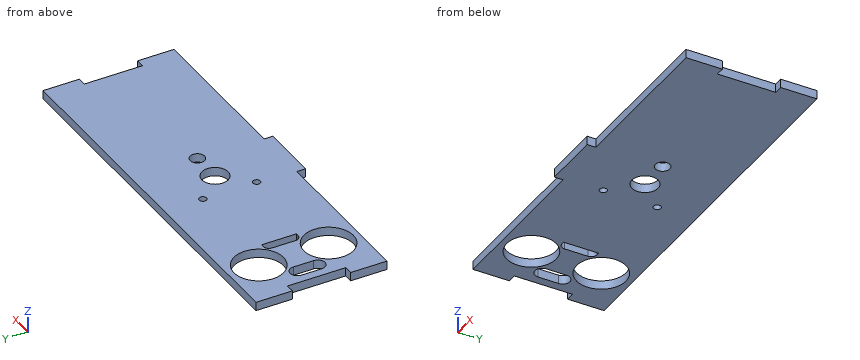
from build123d import *

# Parameters (mm, degrees)
SKETCH1_R           = 8.5
SKETCH1_R_2         = 4.5
SKETCH1_R_3         = 2.5
SKETCH1_R_4         = 1.25
BOSS_EXTRUDE1_DEPTH = 3


with BuildPart() as part:
    # Sketch1 → Boss-Extrude1 (new body)
    with BuildSketch(Plane.XY):
        Polygon((-10, -22.5), (-65, -22.5), (-65, -10), (-62, -10), (-62, 10), (-65, 10), (-65, 22.5), (65, 22.5), (65, 10), (62, 10), (62, -10), (65, -10), (65, -22.5), (10, -22.5), (10, -25.5), (-10, -25.5), align=None)
        with Locations((-48, 12)):
            Circle(SKETCH1_R, mode=Mode.SUBTRACT)
        with Locations((-48, -12)):
            Circle(SKETCH1_R, mode=Mode.SUBTRACT)
        Circle(SKETCH1_R_2, mode=Mode.SUBTRACT)
        with Locations((10.75, 0)):
            Circle(SKETCH1_R_3, mode=Mode.SUBTRACT)
        with Locations((-9, 9.25)):
            Circle(SKETCH1_R_4, mode=Mode.SUBTRACT)
        with Locations(Location((-9, -9.25, 0), (0, 0, 180))):
            Circle(SKETCH1_R_4, mode=Mode.SUBTRACT)
        with BuildLine():
            Line((-54, 3.5), (-54, -3.5))
            ThreePointArc((-54, -3.5), (-56.5, -6), (-59, -3.5))
            Line((-59, -3.5), (-59, 3.5))
            ThreePointArc((-59, 3.5), (-56.5, 6), (-54, 3.5))
        make_face(mode=Mode.SUBTRACT)
        with BuildLine():
            Line((-39, -6), (-40, -6))
            ThreePointArc((-40, -6), (-41.414213562, -5.414213562), (-42, -4))
            Line((-42, -4), (-42, 4))
            ThreePointArc((-42, 4), (-41.414213562, 5.414213562), (-40, 6))
            Line((-40, 6), (-39, 6))
            Line((-39, 6), (-39, -6))
        make_face(mode=Mode.SUBTRACT)
    extrude(amount=BOSS_EXTRUDE1_DEPTH)


solid = part.part
Geometry: final body of the model. Coordinates: model frame, mm. Coordinates: 2 decimals unless noted, no trailing zeros. Order: outer loops, then holes, each group sorted by start corner. A loop starts at its lowest first (then second) coordinate and runs counter-clockwise, first axis right, second up.
(1) Section query C-C (x = -48). Return the cut outline in (y, z).
(2) Material intervals for probe 1 along Y at (x, z) = (-48, 2.1); probe 2 along Y at (x, z) = (-9, 1); probe 3 along Y at (x, z) = (10.75, 1.2), sorted ascending.
(3) Section query B-B (z = 0.5). State how many separate pieces and enclosed holes the cut face has, plus the area to 3 significant figures.
(4) Section query A-A (y = -16). Return the cut outline in (x, z), plus the area to 3 significant figures.
(5) First-contact query: pin 1 (0.9 mm diameter, centred on x = -64, z = 1.5, fed in from -Y); pin 2 (1.5 mm diameter, centred on y = -1.5, z = 1, fed in from +X); pin 3 (0.9 mm diameter, centred on y = 1, z = 2, fed in from -X). Flat tips, straight axial feed; report the tip coordinate or a pass-through.
(6) Section query D-D (x = 11.5). Return the cut outline in (y, z).
Solution:
1. outline: (-22.5, 0) - (-20.5, 0) - (-20.5, 3) - (-22.5, 3) - close; (-3.5, 0) - (3.5, 0) - (3.5, 3) - (-3.5, 3) - close; (20.5, 0) - (22.5, 0) - (22.5, 3) - (20.5, 3) - close
2. probe 1: y = -22.5 to -20.5, -3.5 to 3.5, 20.5 to 22.5
2. probe 2: y = -25.5 to -10.5, -8 to 8, 10.5 to 22.5
2. probe 3: y = -22.5 to -2.5, 2.5 to 22.5
3. separate pieces: 1
3. enclosed holes: 8
3. area: 5,150 mm2
4. outline: (-65, 0) - (-55.5, 0) - (-55.5, 3) - (-65, 3) - close; (-40.5, 0) - (65, 0) - (65, 3) - (-40.5, 3) - close
4. area: 345 mm2
5. pin 1: stops at y = -22.5
5. pin 2: stops at x = 62
5. pin 3: stops at x = -62
6. outline: (-22.5, 0) - (-2.38, 0) - (-2.38, 3) - (-22.5, 3) - close; (2.38, 0) - (22.5, 0) - (22.5, 3) - (2.38, 3) - close
